Source: three-view drawing plus pictorial views. Frame: mm from the lowest corner of the part. Round coordinates to 2 decimals unless told otherwise and drop trailing zeros. Loops run counter-clockwise (first coordinate to the right, second up) from the corner with the lowest first, then second, coordinate; pieces in that order, holes last. Notation, with made-up numbers: (14.5, 60) -> (42.5, 60) arc R23 cw to (42.5, 82) -> close; hole circle Ø4 at (19.25, 26). An arc over 180 degrees is marked (long way). Answer as a JSON object with one key per item and string values. Group by question number.
Item 1: Pin query (flat end, axial travel): pin 1 (3.5 mm diameter, centred on x = 1.8, y = 1.8, fed in from -Z); pin 2 (2 mm diameter, centred on x = 15.5, z = 3.5, fed in from -Y); pin 3 (2 mm diameter, centred on y = 7.5, z = 3.5, fed in from +X). Return the tip coordinate at first contact, or that it passes through.
Item 2: Section query C-C on z = 0.35. Return loops of the section in (x, y).
Item 3: Section query D-D on y = 18.6. Return loops of the section in (x, z), and give its area (3 significant figures).
Item 4: Section query B-B on y = 1.8. Return loops of the section in (x, z).
Item 5: Material intervals for line 1 (Y direction, x = 1.8, z = 3.1); line 2 (Z direction, x = 18.25, y = 18.25); line 3 (X direction, y = 5, z = 2.25), sorted ascending. Write a range as [from, to].
Item 6: Section query A-A on x = 1.8. Return loops of the section in (y, z), and give its area (3 significant figures).
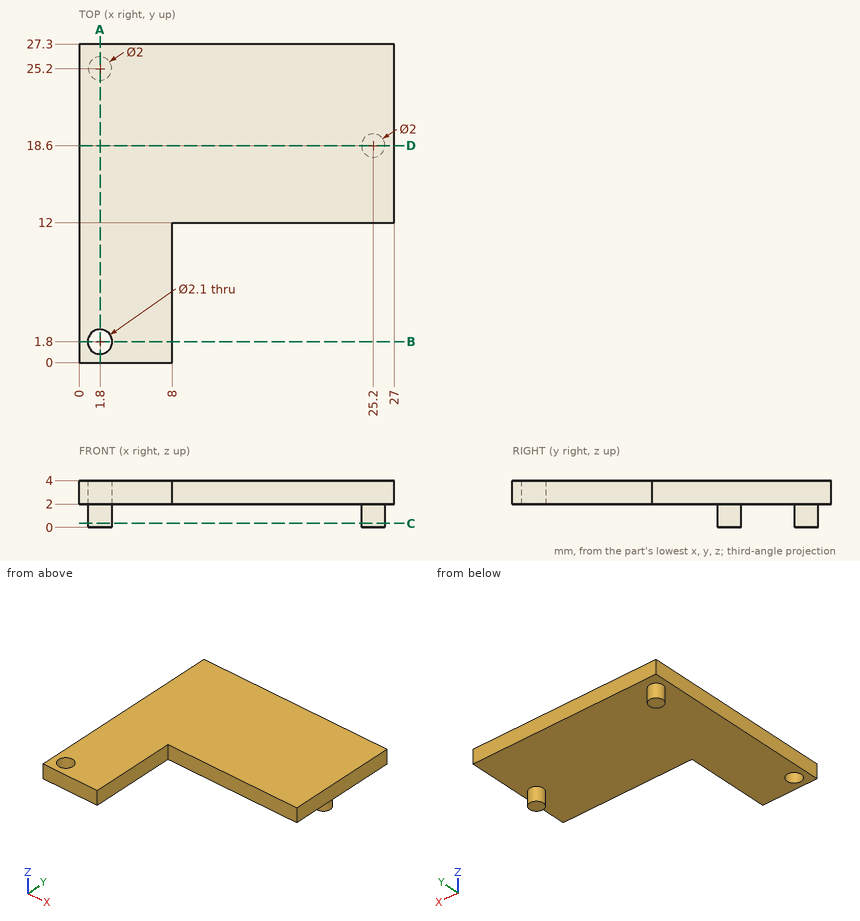
Solved:
{
 "1": {"pin 1": "z = 2", "pin 2": "y = 12", "pin 3": "x = 8"},
 "2": {"outline": "circle Ø2 at (1.8, 25.2); circle Ø2 at (25.2, 18.6)"},
 "3": {"outline": "(0, 2) -> (24.2, 2) -> (24.2, 0) -> (26.2, 0) -> (26.2, 2) -> (27, 2) -> (27, 4) -> (0, 4) -> close", "area": "58.0 mm²"},
 "4": {"outline": "(0, 2) -> (0.75, 2) -> (0.75, 4) -> (0, 4) -> close; (2.85, 2) -> (8, 2) -> (8, 4) -> (2.85, 4) -> close"},
 "5": {"line 1": "[0, 0.75], [2.85, 27.3]", "line 2": "[2, 4]", "line 3": "[0, 8]"},
 "6": {"outline": "(0, 2) -> (0.75, 2) -> (0.75, 4) -> (0, 4) -> close; (2.85, 2) -> (24.2, 2) -> (24.2, 0) -> (26.2, 0) -> (26.2, 2) -> (27.3, 2) -> (27.3, 4) -> (2.85, 4) -> close", "area": "54.4 mm²"}
}
